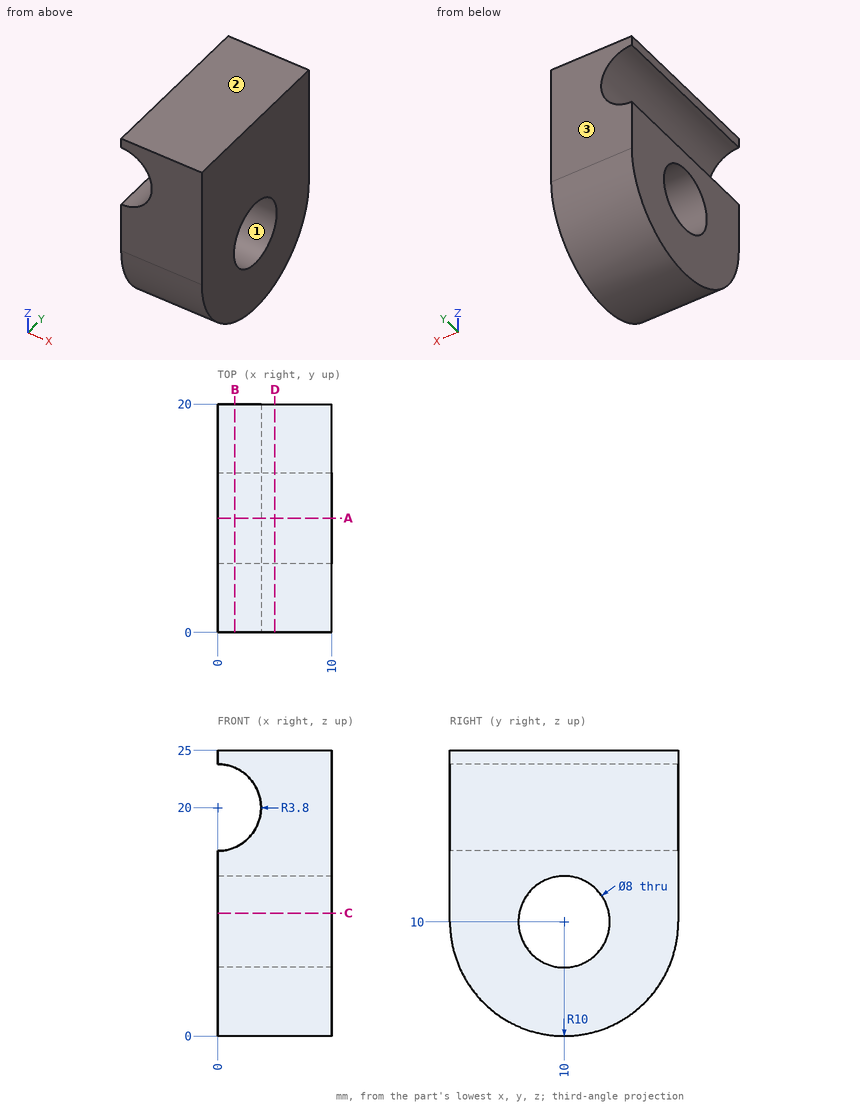
Geometry: see drawing. Coordinates: mm, zero at the bounding-box minimum. Coordinates: 2 decimals unless noted, no trailing zeros. Loops run counter-clockwise (first coordinate to the right, second up) from the corner with the lowest first, then second, coordinate; pieces in that order, holes last. Notation, with made-up numbers: (47.25, -27) - (96.25, -27) arc R24 cw to (96.25, -10) - close; hole circle Ø9 at (-12.75, 35). An arc over 180 degrees is marked (long way). Answer in a Markdown table with one row per item.
(1) Cut plane B-B on x = 1.5. Output: boundary loops of the cut face in (y, z), plus the area to 3 significant figures.
Model answer:
| item | result |
|---|---|
| outline | (0, 10) arc R10 ccw to (20, 10) - (20, 16.51) - (0, 16.51) - close; (0, 23.49) - (20, 23.49) - (20, 25) - (0, 25) - close; hole circle Ø8 at (10, 10) |
| area | 267 mm² |
(2) Cut plane C-C on z = 10.75. Output: boundary loops of the cut face in (x, y), plus the area to 3 significant figures.
Model answer:
| item | result |
|---|---|
| outline | (0, 0) - (10, 0) - (10, 6.07) - (0, 6.07) - close; (0, 13.93) - (10, 13.93) - (10, 20) - (0, 20) - close |
| area | 121 mm² |
(3) Mould query, pull axis Z, two halves, no side actions, for the marked faces 1, 2 and 3. Classes: pulls with the +Z half, pulls with the -Z half, needs draft (parallel to the pull), parting line crosses it, or undercut.
Model answer:
| item | result |
|---|---|
| face 1 | undercut |
| face 2 | pulls with the +Z half |
| face 3 | needs draft |
(4) Material intervals for L1, parallel to Z at x = 2.25, y = 7.5; L2, parallel to Z at x = 5.75, y = 10; L3, parallel to Z at x = 2.25, y = 11.5, sorted ascending. Write a range as from..to.
Model answer:
| item | result |
|---|---|
| L1 | z = 0.32..6.88, 13.12..16.94, 23.06..25 |
| L2 | z = 0..6, 14..25 |
| L3 | z = 0.11..6.29, 13.71..16.94, 23.06..25 |
(5) Pin query (flat end, axial travel): P1, Ø4, axis at x = 3.5, y = 15.5, coming from the -Z side; P2, Ø1, axis at x = 1, y = 12.5, coming from the -Z side; P3, Ø6, axis at x = 8.5, z = 3, coming from the +Y side. Return the tip coordinate at first contact, or that it passes through.
Model answer:
| item | result |
|---|---|
| P1 | stops at z = 0.63 |
| P2 | stops at z = 0.2 |
| P3 | stops at y = 19.17 |
(6) Cut plane A-A on y = 10. Output: boundary loops of the cut face in (x, z), plus the area to 3 significant figures.
Model answer:
| item | result |
|---|---|
| outline | (0, 0) - (10, 0) - (10, 6) - (0, 6) - close; (0, 14) - (10, 14) - (10, 25) - (0, 25) - (0, 23.8) arc R3.8 cw to (0, 16.2) - close |
| area | 147 mm² |
(7) Cut plane D-D on x = 5. Output: boundary loops of the cut face in (y, z).
Model answer:
| item | result |
|---|---|
| outline | (0, 10) arc R10 ccw to (20, 10) - (20, 25) - (0, 25) - close; hole circle Ø8 at (10, 10) |
